Geometry: see drawing. Coordinates: mm, zero at the bounding-box minimum. Coordinates: 2 decimals unless noted, no trailing zeros. Loops run counter-clockwise (first coordinate to the right, second up) from the corner with the lowest first, then second, coordinate; pieces in that order, holes last. Notation, with made-up numbers: (28.5, 81.5) -> (40.5, 81.5) arc R18 ccw to (40.5, 104.5) -> close; hole circle Ø4 at (27, 36.5). An arc over 180 degrees is marked (long way). Answer as a JSON object with one key per item and string values.
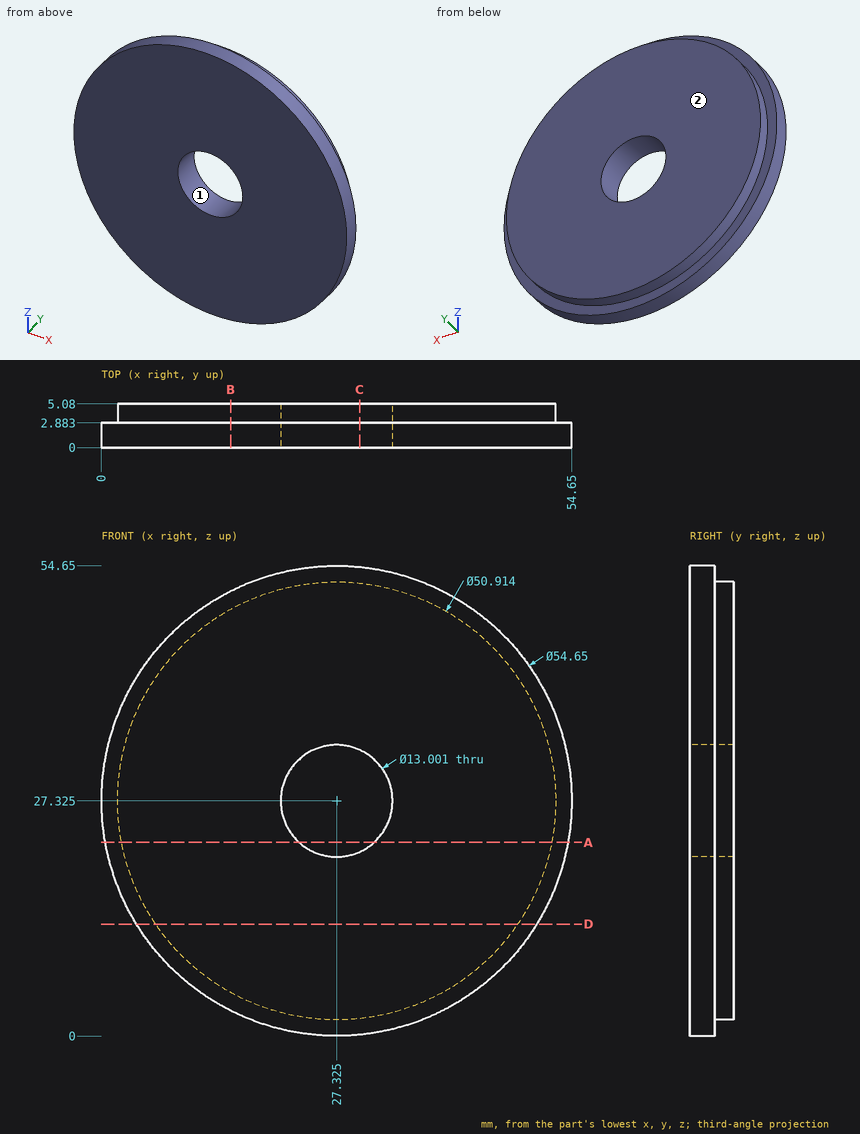
1. Mould query, pull axis Z, two halves, no side actions, for the marked faces 1 and 2. Classes: pulls with the +Z half, pulls with the -Z half, needs draft (parallel to the pull), parting line crosses it, or undercut.
Reply:
{"face 1": "undercut", "face 2": "needs draft"}
2. Line query: line 1 along Y through (x, z) = (16.5, 50.5); line 2 along Z through (x, y) = (21.5, 1.7); line 3 along X through (y, z) = (0.65, 26.5). Output: solid intervals per line, ascending.
Reply:
{"line 1": "y = 0 to 2.88", "line 2": "z = 0.63 to 24.44, 30.21 to 54.02", "line 3": "x = 0.01 to 20.88, 33.77 to 54.64"}
3. Section query D-D (z = 13). Return loops of the section in (x, y).
Reply:
{"outline": "(4.06, 0) -> (50.59, 0) -> (50.59, 2.88) -> (48.37, 2.88) -> (48.37, 5.08) -> (6.28, 5.08) -> (6.28, 2.88) -> (4.06, 2.88) -> close"}
4. Pin query (flat end, axial travel): P1, Ø10, axis at x = 39.5, z = 46.5, coming from the -Y side; P2, Ø1, axis at y = 4.5, z = 29.5, coming from the -X side; P3, Ø2, axis at x = 6.5, z = 8.5, coming from the +Y side; P4, Ø8, axis at x = 27.325, z = 27.325, coming from the -Y side. Return the tip coordinate at first contact, or that it passes through.
Reply:
{"P1": "stops at y = 0", "P2": "stops at x = 1.92", "P3": "stops at y = 2.88", "P4": "passes through"}
5. Section query A-A (z = 22.5). Return loops of the section in (x, y).
Reply:
{"outline": "(0.43, 0) -> (22.97, 0) -> (22.97, 5.08) -> (2.33, 5.08) -> (2.33, 2.88) -> (0.43, 2.88) -> close; (31.68, 0) -> (54.22, 0) -> (54.22, 2.88) -> (52.32, 2.88) -> (52.32, 5.08) -> (31.68, 5.08) -> close"}
6. Section query B-B (x = 15). Return loops of the section in (y, z).
Reply:
{"outline": "(0, 2.94) -> (2.88, 2.94) -> (2.88, 5.05) -> (5.08, 5.05) -> (5.08, 49.6) -> (2.88, 49.6) -> (2.88, 51.71) -> (0, 51.71) -> close"}
7. Section query C-C (x = 30). Return loops of the section in (y, z).
Reply:
{"outline": "(0, 0.13) -> (2.88, 0.13) -> (2.88, 2.01) -> (5.08, 2.01) -> (5.08, 21.4) -> (0, 21.4) -> close; (0, 33.25) -> (5.08, 33.25) -> (5.08, 52.64) -> (2.88, 52.64) -> (2.88, 54.52) -> (0, 54.52) -> close"}
